Source: CAD feature listing. Evaluate the final solid. Frame: model axes, mm. Face numbers are marked on the shaded views. A direction names the side the tool comes from. Give positions to 0.01 mm unless a question says otherwise; leave off trailing zeros. Loops run counter-clockwise (first coordinate to the right, second up) from the corner with the lowest first, then second, coordinate; pieces in that order, holes last. Notation, with made-up numbers: M 42.25,37.25 L 59.25,37.25 A24 cw 59.25,76.25 Z; hole C -19.5,67 d10. An arc over 180 degrees is marked long. Answer in a Markdown table with one row per item.
```python
from build123d import *

# Parameters (mm, degrees)
SKETCH1_R             = 30
BASE_CORE_DEPTH       = 4
SKETCH2_R             = 22
CLEARNESS_DEPTH       = 1
SKETCH3_R             = 20
BREAING_40_ID_DEPTH   = 7
SKETCH4_R             = 10.5
BREAING_21_OD_DEPTH   = 5
SKETCH5_R             = 10.5
MOTOR_CUT_DEPTH       = 7
M3_TAPPED_HOLE2_D     = 2.5
M3_TAPPED_HOLE2_DEPTH = 6.748924226
M3_TAPPED_HOLE2_TIP   = 0.751075774
M3_TAPPED_HOLE1_D     = 2.5


with BuildPart() as part:
    # Sketch1 → base-core (new body)
    with BuildSketch(Plane(origin=(0, 0, 0), x_dir=(1, 0, 0), z_dir=(0, 1, 0))):
        Circle(SKETCH1_R)
    extrude(amount=-BASE_CORE_DEPTH)

    # Sketch2 → clearness (add)
    with BuildSketch(Plane(origin=(0, 0, 0), x_dir=(1, 0, 0), z_dir=(0, 1, 0))):
        Circle(SKETCH2_R)
    extrude(amount=CLEARNESS_DEPTH)

    # Sketch3 → breaing-40-ID (add)
    with BuildSketch(Plane(origin=(0, 1, 0), x_dir=(1, 0, 0), z_dir=(0, 1, 0))):
        Circle(SKETCH3_R)
    extrude(amount=BREAING_40_ID_DEPTH)

    # Sketch4 → breaing-21-OD (cut)
    with BuildSketch(Plane(origin=(0, 8, 0), x_dir=(1, 0, 0), z_dir=(0, 1, 0))):
        Circle(SKETCH4_R)
    extrude(amount=-BREAING_21_OD_DEPTH, mode=Mode.SUBTRACT)

    # Sketch5 → motor-cut (cut)
    with BuildSketch(Plane.XZ.offset(4)):
        Circle(SKETCH5_R)
    extrude(amount=-MOTOR_CUT_DEPTH, mode=Mode.SUBTRACT)

    # M3 Tapped Hole2
    with Locations(Plane(origin=(0, 8, 0), x_dir=(1, 0, 0), z_dir=(0, 1, 0))):
        with Locations((12.727922061, 12.727922061), (18, 0), (12.727922061, -12.727922061), (0, -18), (-12.727922061, -12.727922061), (-18, 0), (-12.727922061, 12.727922061), (0, 18), (0, 0)):
            Hole(M3_TAPPED_HOLE2_D / 2, depth=M3_TAPPED_HOLE2_DEPTH)
            with Locations((0, 0, -(M3_TAPPED_HOLE2_DEPTH + M3_TAPPED_HOLE2_TIP / 2))):  # 118° drill point
                Cone(0, M3_TAPPED_HOLE2_D / 2, M3_TAPPED_HOLE2_TIP, mode=Mode.SUBTRACT)

    # M3 Tapped Hole1 (through all)
    with Locations(Plane.XZ.offset(4)):
        with Locations((-26, 0), (0, 26), (26, 0), (0, -26)):
            Hole(M3_TAPPED_HOLE1_D / 2)


solid = part.part
```
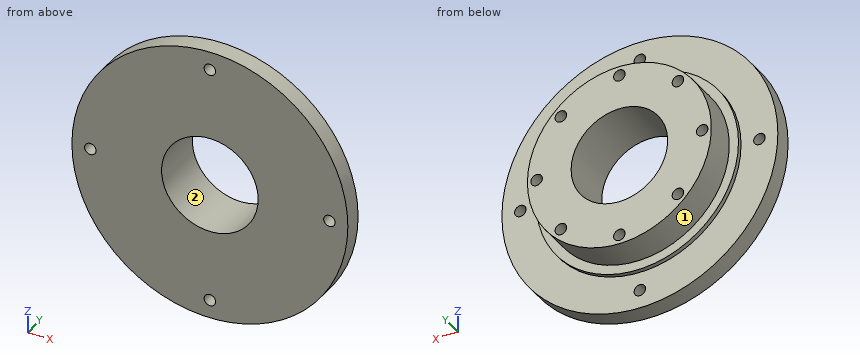
1) Section C-C, the plane y = 6. Count the separate pieces of the cut face and the enclosed holes in it, then the cut area to 3 significant figures.
Reply:
| item | result |
|---|---|
| separate pieces | 1 |
| enclosed holes | 9 |
| area | 871 mm² |
2) Section B-B, the plane z = -26. Return loops of the section in (x, y), then the cut area to 3 significant figures.
Reply:
| item | result |
|---|---|
| outline | M -14.97,-4 L -1.25,-4 L -1.25,0 L -14.97,0 Z; M 1.25,-4 L 14.97,-4 L 14.97,0 L 1.25,0 Z |
| area | 110 mm² |
3) Material intervals for L1, parallel to Z at x = 0, y = 5.25; L2, parallel to Z at x = -1, y = -0.5; L3, parallel to Y at x = 24, z = -11, sorted ascending.
Reply:
| item | result |
|---|---|
| L1 | z = -20 to -19.25, -16.75 to -10.5, 10.5 to 16.75, 19.25 to 20 |
| L2 | z = -29.98 to -26.75, -25.25 to -10.45, 10.45 to 25.25, 26.75 to 29.98 |
| L3 | y = -4 to 0 |
4) Set-up query: the marked faces 1 and 2. Return all of +Z, -Z, +X, -X, +Y, -Y with unobstructed straight access to the full face (end or side cutting, diameter ignored); none if empty.
Reply:
| item | result |
|---|---|
| face 1 | +Y |
| face 2 | +Y, -Y |
5) Pin query (flat end, axial travel): pin 1 Ø4 at (x, y) = (-23, -3) entering from +Z; pin 2 Ø6 at (x, z) = (-21, -18.5) entering from +Y; pin 3 Ø5 at (x, y) = (12.5, -2) entering from -Z; pin 4 Ø1.5 at (x, z) = (0, -26) entering from +Y. Return the tip coordinate at first contact, or that it passes through.
Reply:
| item | result |
|---|---|
| pin 1 | stops at z = 21.42 |
| pin 2 | stops at y = 0 |
| pin 3 | stops at z = -28.28 |
| pin 4 | passes through |
6) Section A-A, the plane x = -8. Return loops of the section in (y, z).
Reply:
| item | result |
|---|---|
| outline | M -4,-28.91 L 0,-28.91 L 0,-20.49 L 1,-20.49 L 1,-18.33 L 8,-18.33 L 8,-6.8 L -4,-6.8 Z; M -4,6.8 L 8,6.8 L 8,18.33 L 1,18.33 L 1,20.49 L 0,20.49 L 0,28.91 L -4,28.91 Z |
7) Section D-D, the plane x = -26. Return loops of the section in (y, z), then the cut area to 3 significant figures.
Reply:
| item | result |
|---|---|
| outline | M -4,-14.97 L 0,-14.97 L 0,-1.25 L -4,-1.25 Z; M -4,1.25 L 0,1.25 L 0,14.97 L -4,14.97 Z |
| area | 110 mm² |
